Geometry check sheet. Reference: the model listing, model coordinates, mm. A direction names the side the tool comes from. Coordinates: 2 decimals unless noted, no trailing zeros. Write each loop counter-clockwise with the first axis right and the second up, starting at its lowest first coordinate (ties: lowest second). Pieces come first, ordered by that corner, then holes. Notation, with made-up numbers: M 42.25,1 L 65.25,1 A22 cw 65.25,13 Z; hole C 50,45 d10. An arc over 180 degrees is marked long. Answer as a JSON object with one key per item and string values. Group by question number.
Autodesk Inventor part; units mm, degrees
sketch "Skizze1" plane through (0, 0, 0) normal (0, 0, 1) x (1, 0, 0)
  line L0 (-33, 46) -> (33, 46)
  line L1 (33, 46) -> (33, -46)
  line L2 (33, -46) -> (-33, -46)
  line L3 (-33, -46) -> (-33, 46)
  line L4 (0, -64.4) -> (0, 64.4)
  line L5 (-46.2, 0) -> (46.2, 0)
  point P0 (0, 0)
  dimension "d0" = 66
  dimension "d1" = 92
extrude "Extrusion1" add sketch "Skizze1" along normal blind 37
sketch "Skizze2" plane through (0, 0, 37) normal (0, 0, 1) x (1, 0, 0)
  line L0 (-33, -46) -> (33, -46)
  line L1 (-23, -46) -> (23, -46)
  line L2 (23, -46) -> (23, -16)
  line L3 (23, -16) -> (-23, -16)
  line L4 (-23, -16) -> (-23, -46)
  line L5 (0, -64.4) -> (0, 64.4)
  point P0 (0, 0)
  dimension "d4" = 46
  dimension "d5" = 30
extrude "Extrusion2" cut sketch "Skizze2" against normal blind 37
sketch "Skizze3" plane through (0, 0, 37) normal (0, 0, 1) x (1, 0, 0)
  line L0 (33, 46) -> (-33, 46)
  line L1 (-29, 46) -> (29, 46)
  line L2 (29, 46) -> (29, -12)
  line L3 (29, -12) -> (-29, -12)
  line L4 (-29, -12) -> (-29, 46)
  line L5 (0, -64.4) -> (0, 64.4)
  point P0 (0, 0)
  dimension "d8" = 58
  dimension "d9" = 58
extrude "Extrusion3" cut sketch "Skizze3" against normal blind 33
sketch "Skizze9" plane through (33, -46, 0) normal (1, 0, 0) x (0, 0, -1)
  line L0 (-18.5, 4.5) -> (-18.5, 28.5) construction
  line L1 (-16.5, 4.5) -> (-16.5, 28.5)
  line L2 (-20.5, 28.5) -> (-20.5, 4.5)
  arc A0 (-20.5, 4.5) -> (-16.5, 4.5) centre (-18.5, 4.5) ccw
  arc A1 (-16.5, 28.5) -> (-20.5, 28.5) centre (-18.5, 28.5) ccw
  line L3 (0, 0) -> (-37, 0)
  line L4 (0, 0) -> (0, 92)
  line L5 (-30.5, 16.5) -> (-6.5, 16.5) construction
  line L6 (-30.5, 14.5) -> (-6.5, 14.5)
  line L7 (-6.5, 18.5) -> (-30.5, 18.5)
  arc A2 (-30.5, 18.5) -> (-30.5, 14.5) centre (-30.5, 16.5) ccw
  arc A3 (-6.5, 14.5) -> (-6.5, 18.5) centre (-6.5, 16.5) ccw
  line L8 (-21.5851, 21.2663) -> (-20.5, 28.5)
  line L9 (-15.4149, 21.2663) -> (-16.5, 28.5)
  line L10 (-21.5851, 11.7337) -> (-20.5, 4.5)
  line L11 (-15.4149, 11.7337) -> (-16.5, 4.5)
  line L12 (-23.2663, 19.5851) -> (-30.5, 18.5)
  line L13 (-23.2663, 13.4149) -> (-30.5, 14.5)
  line L14 (-13.7337, 19.5851) -> (-6.5, 18.5)
  line L15 (-13.7337, 13.4149) -> (-6.5, 14.5)
  arc A4 (-23.2663, 19.5851) -> (-21.5851, 21.2663) centre (-23.5629, 21.5629) ccw
  arc A5 (-15.4149, 21.2663) -> (-13.7337, 19.5851) centre (-13.4371, 21.5629) ccw
  arc A6 (-13.7337, 13.4149) -> (-15.4149, 11.7337) centre (-13.4371, 11.4371) ccw
  arc A7 (-21.5851, 11.7337) -> (-23.2663, 13.4149) centre (-23.5629, 11.4371) ccw
  point P0 (0, 46)
  point P1 (-18.5, 16.5)
  point P2 (-18.5, 16.5)
  point P3 (-22, 18.5)
  point P4 (-15, 18.5)
  point P5 (-22, 14.5)
  point P6 (-15, 14.5)
  point P7 (-20.5, 20)
  point P8 (-20.5, 13)
  point P9 (-16.5, 20)
  point P10 (-16.5, 13)
  point P11 (-20.5, 4.5)
  point P12 (-16.5, 4.5)
  dimension "d59" = 4.5
  dimension "d60" = 2
  dimension "d62" = 4
  dimension "d63" = 24
  dimension "d65" = 24
  dimension "d66" = 2
extrude "Extrusion5" cut sketch "Skizze9" against normal blind 3
properties part number "Block"
1) Section check D-D (z = 18.5). Record the cut outline in (x, y).
2) Set-up check for faces 1 (the flat face through (29, 17, 21)), 2 (the cylindrical face through (31.5, -43.5, 18.5)), 3 (the flat face through (33, 1, 18)), 4 (the flat face through (23, -31, 19)): record each of +Z, -Z, +X, -X, +Y, -Y from which the full face is reachable in a straight line by a thin tool's end or side.
3) Section check A-A (y = -29.5). Record the cut outline in (x, z).
4) Go/stop test with flat-tipped pins: pin 1 Ø16.5 at (x, z) = (4.5, 18) entering from +Y; pin 2 Ø12 at (x, y) = (6.5, 16) entering from +Z; pin 3 Ø5 at (x, z) = (-18, 25.5) entering from -Y. Record where each tip stops, or that it passes through.
5) Section check C-C (x = -3.5). Record the cut outline in (y, z).
6) Draft check along Z on faces 5 (the flat face through (31.52, -26.95, 10.17)), 6 (the flat face through (-33, -1, 18)). Enter one of: +Z half, -Z half, draft (parallel to the pull), parting line (faces both ways), or undercut.
7) Material ranges on probe 1 along X at (y, z) = (-38.5, 8); probe 2 along X at (y, z) = (25.5, 33.5); probe 3 along Z at (x, y) = (24, 40.5), recorded low to high. Write a range as [from, to].
8) Section check B-B (y = -11). Record the cut outline in (x, z), then the cut area to 3 significant figures.
Entries:
{
 "1": {"outline": "M -33,-46 L -23,-46 L -23,-16 L 23,-16 L 23,-46 L 33,-46 L 33,-43.5 L 30,-43.5 L 30,-15.5 L 33,-15.5 L 33,46 L 29,46 L 29,-12 L -29,-12 L -29,46 L -33,46 Z"},
 "2": {"face 1": "+Z, +Y", "face 2": "+X", "face 3": "+Z, -Z, +X, +Y, -Y", "face 4": "+Z, -Z, -Y"},
 "3": {"outline": "M -33,0 L -23,0 L -23,37 L -33,37 Z; M 23,0 L 33,0 L 33,4.5 L 30,4.5 L 30,32.5 L 33,32.5 L 33,37 L 23,37 Z"},
 "4": {"pin 1": "y = -12", "pin 2": "z = 4", "pin 3": "y = -16"},
 "5": {"outline": "M -16,0 L 46,0 L 46,4 L -12,4 L -12,37 L -16,37 Z"},
 "6": {"face 5": "undercut", "face 6": "draft"},
 "7": {"probe 1": "[-33, -23], [23, 33]", "probe 2": "[-33, -29], [29, 33]", "probe 3": "[0, 4]"},
 "8": {"outline": "M -33,0 L 33,0 L 33,37 L 29,37 L 29,4 L -29,4 L -29,37 L -33,37 Z", "area": "528 mm^2"}
}
